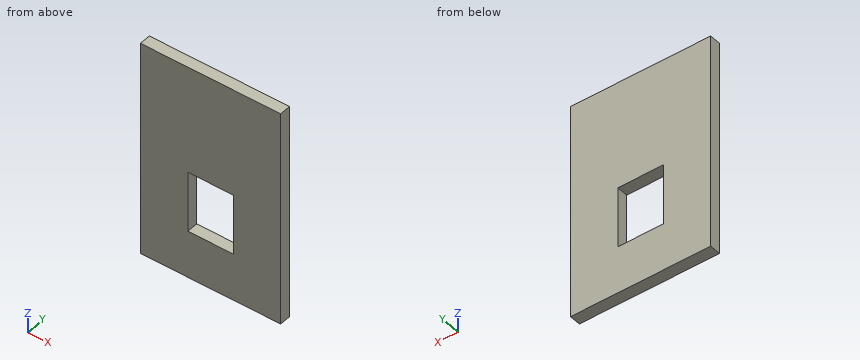
from build123d import *

# Parameters (mm, degrees)
F6_W     = 185
F6_H     = 285
F7_DEPTH = 15
F8_W     = 60
F8_H     = 80
F9_DEPTH = 15


with BuildPart() as f7:
    # F6 (on offset) → F7 (new body, through all)
    with BuildSketch(Plane.XZ.offset(-150)):
        with Locations((0, 150)):
            Rectangle(F6_W, F6_H)
    extrude(amount=F7_DEPTH)

    # F8 (on offset) → F9 (cut, through all)
    with BuildSketch(Plane.XZ.offset(-150)):
        with Locations((0, 110)):
            Rectangle(F8_W, F8_H)
    extrude(amount=F9_DEPTH, mode=Mode.SUBTRACT)


solid = f7.part
Work out the finished part from the listing and answer in its coordinate system (mm). Give positions to 0.01 mm unless a question says otherwise; leave off trailing zeros. Order: outer loops, then holes, each group sorted by start corner. A loop starts at its lowest first (then second) coordinate and runs counter-clockwise, first axis right, second up. Notation, with made-up numbers: (22.5, 62.25) -> (77.5, 62.25) arc R4 ccw to (77.5, 66.25) -> close; hole circle Ø3 at (-23.75, -16). An arc over 180 degrees is marked (long way). One line per item, written item: value.
Item 1: Find section B-B, the plane y = 142.5. Give the vertices of the cut face in (x, z).
Answer sheet:
outline: (-92.5, 7.5) -> (92.5, 7.5) -> (92.5, 292.5) -> (-92.5, 292.5) -> close; hole (-30, 70) -> (30, 70) -> (30, 150) -> (-30, 150) -> close
Item 2: Find section A-A, the plane x = 20.5. Give the vertices of the cut face in (y, z).
Answer sheet:
outline: (135, 7.5) -> (150, 7.5) -> (150, 70) -> (135, 70) -> close; (135, 150) -> (150, 150) -> (150, 292.5) -> (135, 292.5) -> close
Item 3: Straight lines are drawn through the part: probe 1 along Z at (x, y) = (-1.5, 143.5); probe 2 along X at (y, z) = (148.75, 93.5). For each, find the intervals that lie inside material, in ascending order.
Answer sheet:
probe 1: 7.5 to 70, 150 to 292.5
probe 2: -92.5 to -30, 30 to 92.5
Item 4: Find section C-C, the plane z = 103.5. Give the vertices of the cut face in (x, y).
Answer sheet:
outline: (-92.5, 135) -> (-30, 135) -> (-30, 150) -> (-92.5, 150) -> close; (30, 135) -> (92.5, 135) -> (92.5, 150) -> (30, 150) -> close
